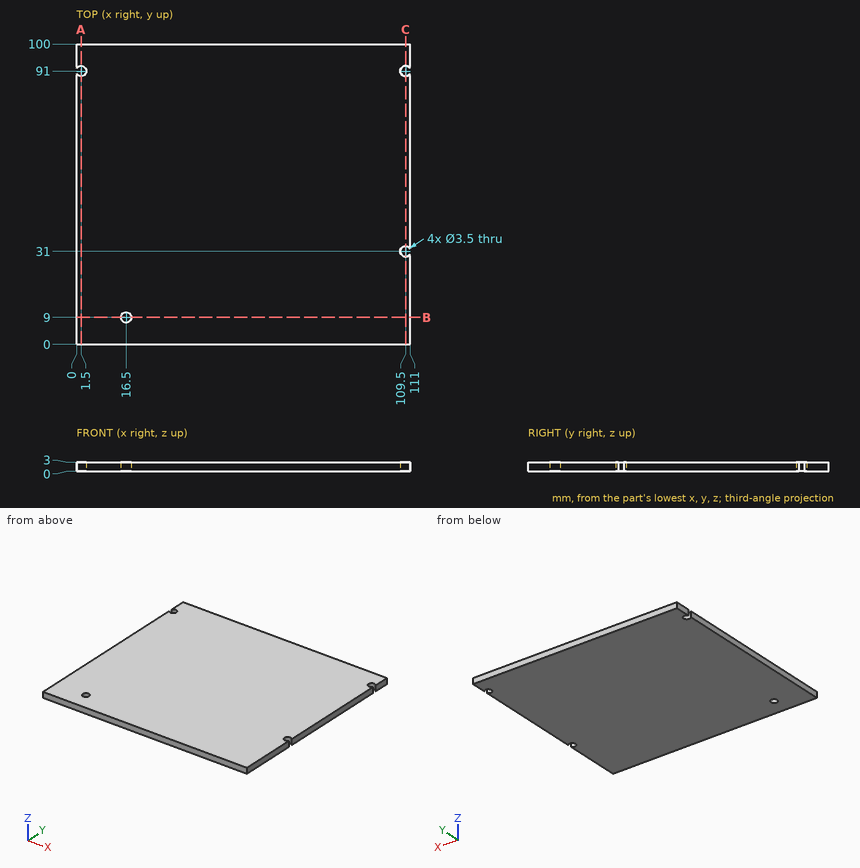
Geometry check sheet. Reference: drawing and pictorial views, mm from the part's lowest x, y, z. Coordinates: 2 decimals unless noted, no trailing zeros. Order: outer loops, then holes, each group sorted by start corner. A loop starts at its lowest first (then second) coordinate and runs counter-clockwise, first axis right, second up.
Item 1: Section check A-A (x = 1.5). Enter the section's corners in (y, z).
Item 2: Section check B-B (y = 9). Enter the section's corners in (x, z).
Item 3: Scan lines: line 1 along Y through (x, z) = (109.5, 1.7); line 2 along Y through (x, z) = (16.5, 0.95); line 3 along Y through (x, z) = (1.5, 2). Record each from-to range of solid material in increasing order.
Item 4: Section check C-C (x = 109.5). Enter the section's corners in (y, z).
Check sheet entries:
1. outline: (0, 0) - (89.25, 0) - (89.25, 3) - (0, 3) - close; (92.75, 0) - (100, 0) - (100, 3) - (92.75, 3) - close
2. outline: (0, 0) - (14.75, 0) - (14.75, 3) - (0, 3) - close; (18.25, 0) - (111, 0) - (111, 3) - (18.25, 3) - close
3. line 1: y = 0 to 29.25, 32.75 to 89.25, 92.75 to 100
3. line 2: y = 0 to 7.25, 10.75 to 100
3. line 3: y = 0 to 89.25, 92.75 to 100
4. outline: (0, 0) - (29.25, 0) - (29.25, 3) - (0, 3) - close; (32.75, 0) - (89.25, 0) - (89.25, 3) - (32.75, 3) - close; (92.75, 0) - (100, 0) - (100, 3) - (92.75, 3) - close
